Job drawing, mm, ordinate dimensions from the low corner. One solid piece. A direction names the side the tool comes from. Give positions to 0.01 mm unless a question says otherwise; leave off trailing zeros. Loops run counter-clockwise (first coordinate to the right, second up) from the corner with the lowest first, then second, coordinate; pieces in that order, holes last. Notation, with made-up numbers: M 14.25,38.25 L 49.25,38.25 A28 cw 49.25,67.25 Z; hole C -17.5,2.5 d7. An arc over 180 degrees is marked long. Put each result on its own line as item: value.
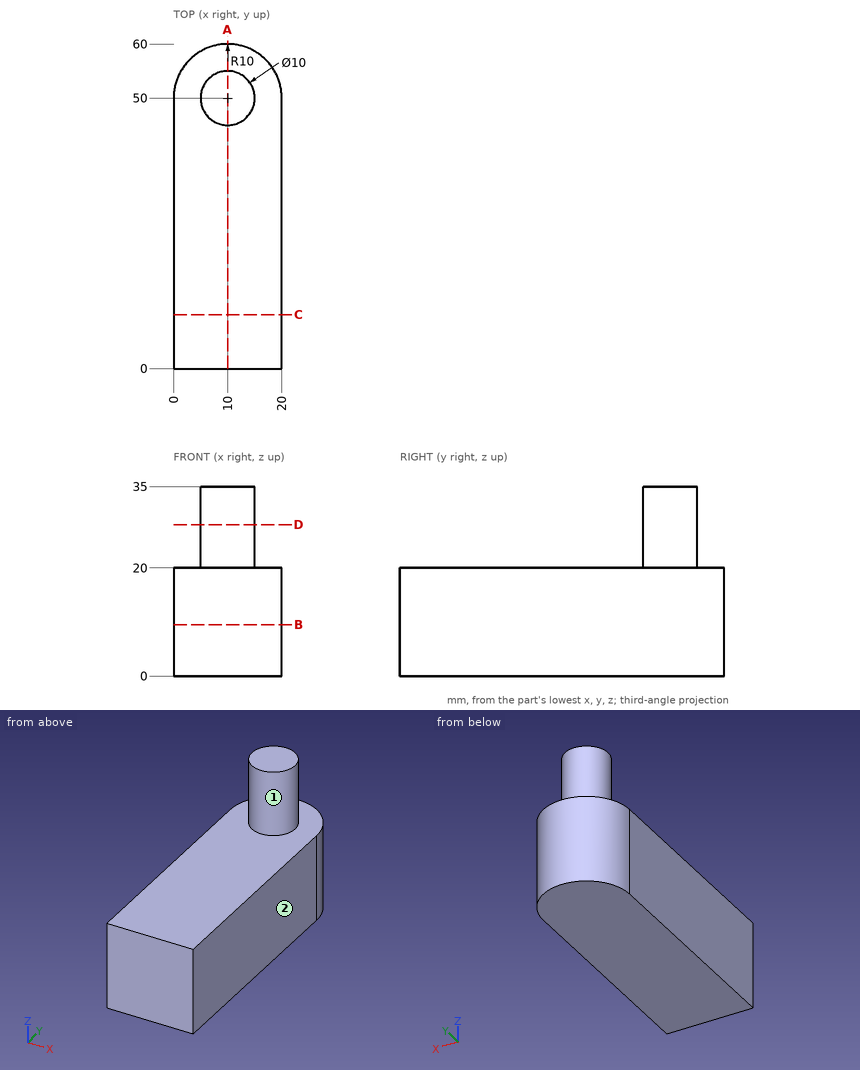
Q1. Slice it at D-D (z = 28). List the corners of the cut face in (x, y).
Here are the results:
outline: C 10,50 d10
Q2. Drop flat-ended pins along their axis: pin 1 Ø5 at (x, z) = (7.5, 23.5) entering from -Y; pin 2 Ø12 at (x, y) = (5.5, 7) entering from +Z; pin 3 Ø2 at (x, z) = (3, 24.5) entering from +Y. Give the stop position or say it passes through.
Here are the results:
pin 1: y = 45
pin 2: z = 20
pin 3: through
Q3. Slice it at C-C (y = 10). List the corners of the cut face in (x, z).
Here are the results:
outline: M 0,0 L 20,0 L 20,20 L 0,20 Z
Q4. Probe line 1 (Z direction, x = 9, y = 16); line 2 (Y direction, x = 7.75, z = 19); line 3 (Y direction, x = 5.5, z = 26). List the from-to ranges inside material, lowest first. Write a range as from..to.
Here are the results:
line 1: 0..20
line 2: 0..59.74
line 3: 47.82..52.18
Q5. Slice it at B-B (z = 9.5). List the corners of the cut face in (x, y).
Here are the results:
outline: M 0,0 L 20,0 L 20,50 A10 ccw 0,50 Z
Q6. Slice it at A-A (x = 10). List the corners of the cut face in (y, z), and give its area (3 significant figures).
Here are the results:
outline: M 0,0 L 60,0 L 60,20 L 55,20 L 55,35 L 45,35 L 45,20 L 0,20 Z
area: 1,350 mm²
Q7. Tool access for the marked faces 1 and 2: list every direction of +Z, -Z, +X, -X, +Y, -Y with a clear straight run to the whole face (end or side of a thin tool).
Here are the results:
face 1: +Z
face 2: +Z, -Z, +X, +Y, -Y
